```python
from build123d import *

# Parameters (mm, degrees)
F0_R     = 14.2875
F0_R_2   = 7.9375
F0_R_3   = 3.96875
F1_DEPTH = 1.5875
F2_DEPTH = 3.175
F3_R     = 1.016
F4_DEPTH = 0.3175
F5_SIZE  = 0.508


with BuildPart() as f1:
    # F0 (on Top) → F1 (new body)
    with BuildSketch(Plane.XY):
        Circle(F0_R)
        Circle(F0_R_2, mode=Mode.SUBTRACT)
        Circle(F0_R_2)
        Circle(F0_R_3, mode=Mode.SUBTRACT)
        Circle(F0_R_3)
    extrude(amount=-F1_DEPTH)

    # F0 (on Top) → F2 (join)
    with BuildSketch(Plane.XY):
        Circle(F0_R_3)
    extrude(amount=F2_DEPTH)

    # F3
    f3_edges = [f1.edges().sort_by_distance(p)[0] for p in [
        (-14.2875, 0, -1.5875),
    ]]
    fillet(f3_edges, radius=F3_R)

    # F0 (on Top) → F4 (join)
    with BuildSketch(Plane.XY):
        Circle(F0_R_2)
        Circle(F0_R_3, mode=Mode.SUBTRACT)
    extrude(amount=F4_DEPTH)

    # F5
    f5_edges = [f1.edges().sort_by_distance(p)[0] for p in [
        (-3.96875, 0, 3.175),
    ]]
    chamfer(f5_edges, length=F5_SIZE)


solid = f1.part
```
Can you work these out from the model? Positions are in its coordinate system, mm. A direction names the side the tool comes from. Give positions to 0.01 mm unless a question says otherwise; leave off trailing zeros. Loops run counter-clockwise (first coordinate to the right, second up) from the corner with the lowest first, then second, coordinate; pieces in that order, holes last. Notation, with made-up numbers: M 53.5,49.25 L 84.5,49.25 A17 ccw 84.5,54.25 Z; hole C -9.75,9 d4. An arc over 180 degrees is marked long. Use CSV: the item, a comma, the result in double quotes. Start each with the question number.
1. Imagine slicing it at C-C, the plane z = 1.25. Write out the boundary of the cut face in (x, y), plus the area to 3 significant figures.
2. On a 3-axis mill with a long thin cutter (end or side, diameter ignored), from which of +Z, -Z, +X, -X, +Y, -Y can I reach the whole of each face in a straight line? I mean faces 1 (the face through (0, 0, -1.588)), 2 (the face through (-1.72, -7.75, 0.16)). Say none if no direction works.
3. If I drill on L1, parallel to Z at x = 8.75, y = 1.75; L2, parallel to Z at x = -4.5, y = 3; L3, parallel to Y at x = 1.5, z = -0.4, over which ranges is the centre line in solid material (lowest first)?
Response values:
1,outline,"C 0,0 d7.94"
1,area,"49.5 mm^2"
2,face 1,"-Z, +X, -X, +Y, -Y"
2,face 2,"+Z"
3,L1,"-1.59 to 0"
3,L2,"-1.59 to 0.32"
3,L3,"-14.21 to 14.21"
